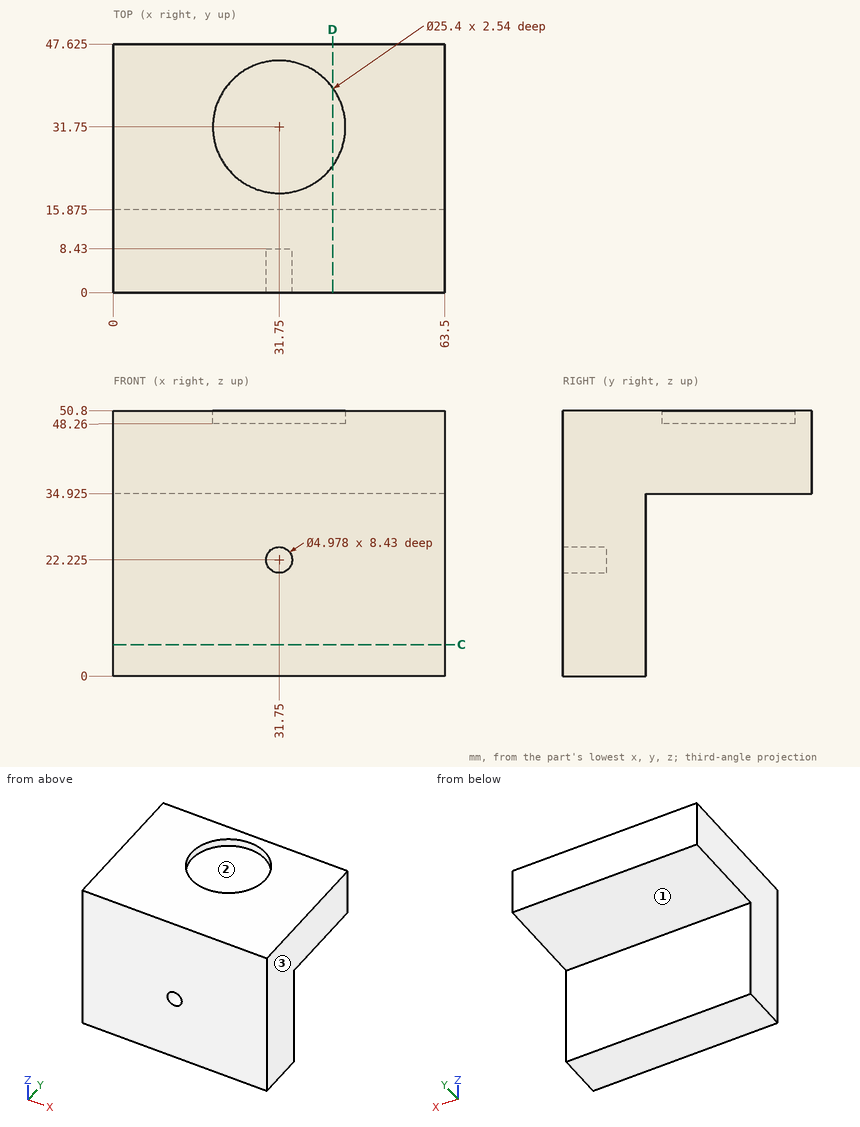
The drawing under review shows one solid part. Ordinate dimensions are in mm from its lowest x, y, z. A direction names the side the tool comes from. Coordinates: 2 decimals unless noted, no trailing zeros. Order: outer loops, then holes, each group sorted by start corner. A loop starts at its lowest first (then second) coordinate and runs counter-clockwise, first axis right, second up. Notation, with made-up numbers: (-3.5, 9) -> (4.5, 9) arc R28 cw to (4.5, 48) -> close; hole circle Ø9 at (6.5, 38). An arc over 180 degrees is marked (long way). Return JSON: item names as keys, results as strings.
1. Machinability: for the marked faces 1, 2 and 3, which of the approach directions +Z, -Z, +X, -X, +Y, -Y give a long, thin tool a straight path to every point of the face, cutting with its end or side? Answer none if there is none.
Answer block:
{"face 1": "-Z, +X, -X, +Y", "face 2": "+Z", "face 3": "+Z, -Z, +X, +Y, -Y"}
2. We need section C-C on z = 6. Write out the cut boundary in (x, y) (1 decimal).
Answer block:
{"outline": "(0, 0) -> (63.5, 0) -> (63.5, 15.9) -> (0, 15.9) -> close"}
3. We need section D-D on x = 42. Write out the cut boundary in (y, z) (1 decimal).
Answer block:
{"outline": "(0, 0) -> (15.9, 0) -> (15.9, 34.9) -> (47.6, 34.9) -> (47.6, 50.8) -> (39.2, 50.8) -> (39.2, 48.3) -> (24.3, 48.3) -> (24.3, 50.8) -> (0, 50.8) -> close"}
4. For pin 1 Ø9.5 at (x, y) = (27, 29.5) entering from -Z (3 decimals); pin 2 Ø1.5 at (x, z) = (39, 15) entering from -Y; pin 3 Ø8 at (x, z) = (31.75, 22.225) entering from +Y (3 decimals); pin 4 Ø1.5 at (x, z) = (30.5, 21.5) entering from -Y, all flat-tipped, find the tip position at first contact; note any pin that passes through.
Answer block:
{"pin 1": "z = 34.925", "pin 2": "y = 0", "pin 3": "y = 15.875", "pin 4": "y = 8.43"}
5. For line 1 (Z direction, x = 31.75, y = 3.75) (1 decimal); line 2 (Y direction, x = 47, z = 12) (1 decimal); line 3 (Z direction, x = 3, y = 26) (1 decimal), list the stretches that pass through material, from the lowest coordinate up. Write a range as from..to.
Answer block:
{"line 1": "0..19.7, 24.7..50.8", "line 2": "0..15.9", "line 3": "34.9..50.8"}
